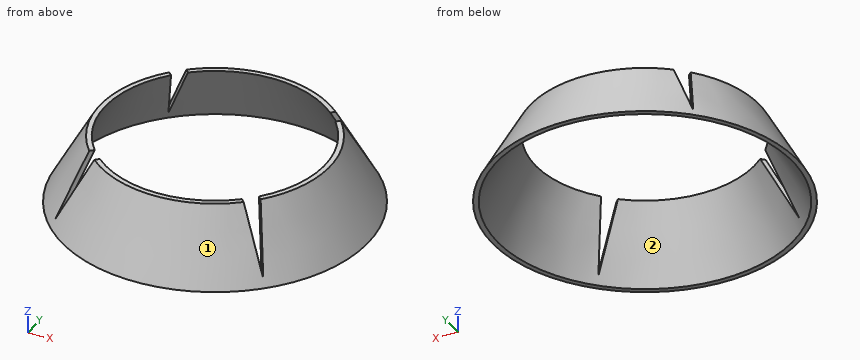
from build123d import *

# Parameters (mm, degrees)
SKETCH018_R           = 58
SKETCH019_R           = 43
SKETCH016_R           = 60
SKETCH017_R           = 45
POCKET003_DEPTH       = 33
POLARPATTERN005_COUNT = 4


with BuildPart() as loft001:
    # Sketch018 → Loft001 section 0
    with BuildSketch(Plane.XY.offset(3)):
        Circle(SKETCH018_R)
    # Sketch019 → Loft001 section 1
    with BuildSketch(Plane.XY.offset(30)):
        Circle(SKETCH019_R)
    loft()


with BuildPart() as support:
    # Sketch016 → Loft section 0
    with BuildSketch(Plane.XY.offset(3)):
        Circle(SKETCH016_R)
    # Sketch017 → Loft section 1
    with BuildSketch(Plane.XY.offset(30)):
        Circle(SKETCH017_R)
    loft()

    # Cut: cut Loft001
    add(loft001.part, mode=Mode.SUBTRACT)

    # Sketch020 → Pocket003 (cut)
    with BuildSketch(Plane(origin=(-50, -50, 0), x_dir=(-0.707107, 0.707107, 0), z_dir=(0.707107, 0.707107, 0))):
        Polygon((0, 6), (-3.748315, 35.090931), (3.748315, 35.090931), align=None)
    pocket003 = extrude(amount=POCKET003_DEPTH, mode=Mode.SUBTRACT)

    # PolarPattern005: Pocket003 ×4 about axis
    polarpattern005_axis = Axis((0, 0, 0), (0, 0, 1))
    for i in range(1, POLARPATTERN005_COUNT):
        add(pocket003.rotate(polarpattern005_axis, i * 360 / POLARPATTERN005_COUNT), mode=Mode.SUBTRACT)


solid = support.part
The listing builds one solid part. Answer for the finished solid, in the listing's coordinates (mm). Face numbers are marked on the shaded views. Coordinates: 2 decimals unless noted, no trailing zeros. Write each loop counter-clockwise with the first axis right and the second up, starting at its lowest first coordinate (ties: lowest second). Pieces come first, ordered by that corner, then holes. Notation, with made-up numbers: (2.25, 5.5) - (25.25, 5.5) arc R10 ccw to (25.25, 13.5) - close; hole circle Ø5 at (-38.75, 24). An arc over 180 degrees is marked (long way). Put each result on its own line as item: value.
1. The part is cut by section C-C on x = -36.5. State how many separate pieces and enclosed holes the cut face has, plus the area to 3 significant figures.
Answer sheet:
separate pieces: 4
enclosed holes: 0
area: 129 mm^2
2. Flat-ended cylindrical pins translate along their axes: pin 1 Ø2 at (y, z) = (4.5, 11.5) entering from -X; pin 2 Ø1.5 at (x, y) = (-31, -42) entering from +Z; pin 3 Ø12 at (y, z) = (-4.5, 15) entering from -X. Find the tip coordinate at first contact, or state that the pin passes through.
Answer sheet:
pin 1: stops at x = -55.66
pin 2: stops at z = 18.39
pin 3: stops at x = -56.52
3. Find the intervals of material crossed by line 1 along X through (y, z) = (9, 28.75); line 2 along Y through (x, z) = (20.5, 18.5); line 3 along Y through (x, z) = (-15, 17.25), in increasing order. Write a range as from..to.
Answer sheet:
line 1: x = -44.8..-42.76, 42.76..44.8
line 2: y = -47.12..-44.93, 44.93..47.12
line 3: y = -49.88..-47.78, 47.78..49.88
4. The part is cut by section A-A on x = 0. Give the vertices of the cut face in (y, z).
Answer sheet:
outline: (-60, 3) - (-58, 3) - (-43, 30) - (-45, 30) - close; (43, 30) - (58, 3) - (60, 3) - (45, 30) - close
5. Determine the mould class of the marked faces 1 and 2 for opening direction X: pulls with the +X half, pulls with the -X half, needs draft (parallel to the pull), parting line crosses it, or undercut.
Answer sheet:
face 1: parting line crosses it
face 2: undercut
6. The part is cut by section B-B on z = 12.5. Give the vertices of the cut face in (x, y).
Answer sheet:
outline: (-39.28, -38.1) - (-37.87, -36.68) arc R52.72 cw to (-37.87, 36.68) - (-39.28, 38.1) arc R54.72 ccw to start; (-38.1, -39.28) arc R54.72 ccw to (38.1, -39.28) - (36.68, -37.87) arc R52.72 cw to (-36.68, -37.87) - close; (-38.1, 39.28) - (-36.68, 37.87) arc R52.72 cw to (36.68, 37.87) - (38.1, 39.28) arc R54.72 ccw to start; (37.87, -36.68) - (39.28, -38.1) arc R54.72 ccw to (39.28, 38.1) - (37.87, 36.68) arc R52.72 cw to start
